Source: CAD feature listing. Evaluate the final solid. Frame: model axes, mm. Give positions to 0.01 mm unless a question says otherwise; leave off trailing zeros. Order: outer loops, then holes, each group sorted by start corner. A loop starts at its lowest first (then second) coordinate and runs counter-clockwise, first axis right, second up.
1) First-contact query: P1, Ø2.5, axis at x = 71.44, z = 123.73, coming from the -Y side; P2, Ø1.5, axis at x = 52, y = 2.5, coming from the +Z side; P3, Ø2, axis at x = -90, y = 1.5, coming from the +Z side. Flat tips, straight axial feed; report the tip coordinate or a pass-through.
2) Section A-A, the plane x = 7.5. Return loops of the section in (y, z).
3) Section B-B, the plane y = 1.7. Give the number of separate pieces and of enclosed holes in the cut face, plus the area to 3 significant figures.
4) Section C-C, the plane z = -168.5. Return loops of the section in (x, y), plus the area to 3 significant figures.
5) Section D-D, the plane x = -88.5. Return loops of the section in (y, z), plus the area to 3 significant figures.
6) Material intervals for line 1 (X direction, y = 2.65, z = -53); line 2 (X direction, y = 3.35, z = -17.78); line 3 (X direction, y = 1.55, z = 71), sorted ascending.
```python
from build123d import *

# Parameters (mm, degrees)
BOSS_EXTRUDE1_DEPTH   = 4.7625
F_8_CLEARANCE_HOLE1_D = 4.4958
CIRPATTERN1_COUNT     = 12
F_4_40_TAPPED_HOLE1_D = 2.2606
CUT_EXTRUDE1_REACH    = 272.048
SKETCH11_W            = 51.189238902
SKETCH11_H            = 119.204570221
CUT_EXTRUDE2_REACH    = 272.048
SKETCH12_W            = 6.35
SKETCH12_H            = 50.8


with BuildPart() as part:
    # Sketch1 → Boss-Extrude1 (new body)
    with BuildSketch(Plane(origin=(0, 0, 0), x_dir=(1, 0, 0), z_dir=(0, 1, 0))):
        with BuildLine():
            Line((177.8, 98.373776994), (177.8, -98.373776994))
            ThreePointArc((177.8, -98.373776994), (0, -203.2), (-177.8, -98.373776994))
            Line((-177.8, -98.373776994), (-177.8, 98.373776994))
            ThreePointArc((-177.8, 98.373776994), (0, 203.2), (177.8, 98.373776994))
        make_face()
    extrude(amount=BOSS_EXTRUDE1_DEPTH)

    # #8 Clearance Hole1 (through all)
    with Locations(Plane(origin=(0, 4.7625, 0), x_dir=(1, 0, 0), z_dir=(0, 1, 0))):
        with Locations((0, -142.875)):
            f_8_clearance_hole1 = Hole(F_8_CLEARANCE_HOLE1_D / 2)

    # CirPattern1: #8 Clearance Hole1 ×12 about axis
    cirpattern1_axis = Axis((0, 0, 0), (0, 1, 0))
    for i in range(1, CIRPATTERN1_COUNT):
        add(f_8_clearance_hole1.rotate(cirpattern1_axis, i * 360 / CIRPATTERN1_COUNT), mode=Mode.SUBTRACT)

    # #4-40 Tapped Hole1 (through all)
    with Locations(Plane(origin=(0, 4.7625, 0), x_dir=(1, 0, 0), z_dir=(0, 1, 0))):
        with Locations((-100.33, 91.5416), (-67.31, 102.9716), (-67.31, 20.32), (-97.79, 17.78), (-100.296230539, -16.186944047), (-67.31, -6.35), (-67.31, -89.0016), (-97.79, -91.5416), (67.31, -102.9716), (100.33, -91.5416), (97.79, -17.78), (67.31, -20.32), (67.31, 6.35), (100.33, 17.78), (97.79, 91.5416), (67.31, 89.0016), (24.13, -22.225), (-24.13, -22.225), (-20.955, -88.265), (20.955, -88.265)):
            Hole(F_4_40_TAPPED_HOLE1_D / 2)

    # Sketch11 → Cut-Extrude1 (cut, up to next)
    with BuildSketch(Plane(origin=(0, 4.7625, 0), x_dir=(1, 0, 0), z_dir=(0, 1, 0)), mode=Mode.PRIVATE) as cut_extrude1_sk1:
        with Locations((0, 64.697510279)):
            Rectangle(SKETCH11_W, SKETCH11_H)
    cut_extrude1_tool1 = extrude(cut_extrude1_sk1.sketch, amount=-CUT_EXTRUDE1_REACH, mode=Mode.PRIVATE) & part.part
    add(cut_extrude1_tool1.solids().sort_by_distance((0, 4.7625, -64.69751))[0], mode=Mode.SUBTRACT)

    # Sketch12 → Cut-Extrude2 (cut, up to next)
    with BuildSketch(Plane(origin=(0, 4.7625, 0), x_dir=(1, 0, 0), z_dir=(0, 1, 0)), mode=Mode.PRIVATE) as cut_extrude2_sk1:
        with Locations((-108.585, 27.94)):
            Rectangle(SKETCH12_W, SKETCH12_H)
    cut_extrude2_tool1 = extrude(cut_extrude2_sk1.sketch, amount=-CUT_EXTRUDE2_REACH, mode=Mode.PRIVATE) & part.part
    # Sketch12 → Cut-Extrude2 (cut, up to next)
    with BuildSketch(Plane(origin=(0, 4.7625, 0), x_dir=(1, 0, 0), z_dir=(0, 1, 0)), mode=Mode.PRIVATE) as cut_extrude2_sk2:
        with Locations((-108.585, -81.3816)):
            Rectangle(SKETCH12_W, SKETCH12_H)
    cut_extrude2_tool2 = extrude(cut_extrude2_sk2.sketch, amount=-CUT_EXTRUDE2_REACH, mode=Mode.PRIVATE) & part.part
    # Sketch12 → Cut-Extrude2 (cut, up to next)
    with BuildSketch(Plane(origin=(0, 4.7625, 0), x_dir=(1, 0, 0), z_dir=(0, 1, 0)), mode=Mode.PRIVATE) as cut_extrude2_sk3:
        with Locations((108.585, 27.94)):
            Rectangle(SKETCH12_W, SKETCH12_H)
    cut_extrude2_tool3 = extrude(cut_extrude2_sk3.sketch, amount=-CUT_EXTRUDE2_REACH, mode=Mode.PRIVATE) & part.part
    # Sketch12 → Cut-Extrude2 (cut, up to next)
    with BuildSketch(Plane(origin=(0, 4.7625, 0), x_dir=(1, 0, 0), z_dir=(0, 1, 0)), mode=Mode.PRIVATE) as cut_extrude2_sk4:
        with Locations((108.585, -81.3816)):
            Rectangle(SKETCH12_W, SKETCH12_H)
    cut_extrude2_tool4 = extrude(cut_extrude2_sk4.sketch, amount=-CUT_EXTRUDE2_REACH, mode=Mode.PRIVATE) & part.part
    add(cut_extrude2_tool1.solids().sort_by_distance((-108.585, 4.7625, -27.94))[0], mode=Mode.SUBTRACT)
    add(cut_extrude2_tool2.solids().sort_by_distance((-108.585, 4.7625, 81.3816))[0], mode=Mode.SUBTRACT)
    add(cut_extrude2_tool3.solids().sort_by_distance((108.585, 4.7625, -27.94))[0], mode=Mode.SUBTRACT)
    add(cut_extrude2_tool4.solids().sort_by_distance((108.585, 4.7625, 81.3816))[0], mode=Mode.SUBTRACT)


solid = part.part
```
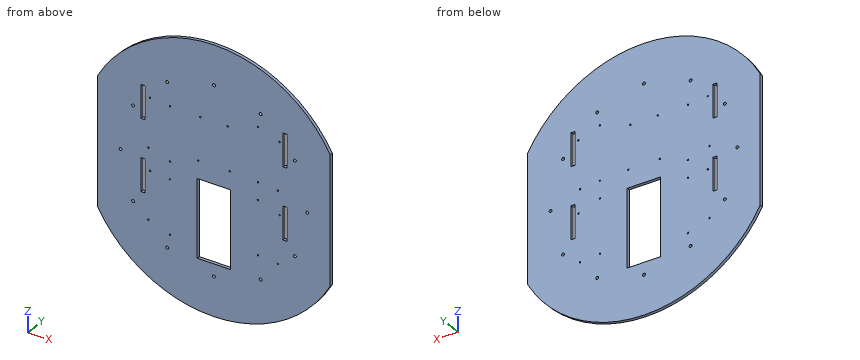
From the geometry:
1. P1: passes through
1. P2: stops at z = 196.63
1. P3: stops at z = 182.67
2. outline: (0, -203.06) - (4.76, -203.06) - (4.76, -124.3) - (0, -124.3) - close; (0, -5.1) - (4.76, -5.1) - (4.76, 203.06) - (0, 203.06) - close
3. separate pieces: 1
3. enclosed holes: 37
3. area: 115,000 mm2
4. outline: (-113.57, 0) - (113.57, 0) - (113.57, 4.76) - (-113.57, 4.76) - close
4. area: 1,080 mm2
5. outline: (0, -182.92) - (4.76, -182.92) - (4.76, 182.92) - (0, 182.92) - close
5. area: 1,740 mm2
6. line 1: x = -177.8 to -111.76, -105.41 to -25.59, 25.59 to 105.41, 111.76 to 177.8
6. line 2: x = -177.8 to -111.76, -105.41 to -98.92, -96.66 to -25.59, 25.59 to 99.2, 101.46 to 105.41, 111.76 to 177.8
6. line 3: x = -177.8 to -125.94, -121.53 to -111.76, -105.41 to 105.41, 111.76 to 121.53, 125.94 to 177.8
